Here's how the part is built. I have some questions about the finished solid (model axes, mm). A direction names the side the tool comes from. Round coordinates to 2 decimals unless told otherwise and drop trailing zeros. Write each loop counter-clockwise with the first axis right and the second up, starting at its lowest first coordinate (ties: lowest second). Pieces come first, ordered by that corner, then holes. Notation, with made-up numbers: M 56,47.25 L 106,47.25 A7 cw 106,59.25 Z; hole C 72,42.5 d10. An arc over 180 degrees is marked long. Use one line per item in the form item = value. Start each with the question number.
Q1. I need wall thicknesses on line 1 along X through (y, z) = (2.2, 14); line 2 along Z through (x, y) = (72, 2.25); line 3 along X through (y, z) = (2.85, 57). Which ranges of each line are inside material? Lowest first, please. Write a range as from..to.
Q2. I want a section at D-D on x = 72. List the corners of the cut face in (y, z) for me, and give its area (3 significant figures).
Q3. I want a section at C-C on z = 14. List the corners of the cut face in (x, y) for me, and give its area (3 significant figures).
Q4. We'd pull the mould along Z, two halves only. Please class faces 6 (the face through (41.243, 9.93, -20.533)), 7 (the face through (28.33, 2.535, 58.617)), 8 (the face through (63, 0, -44)): +Z half, -Z half, draft (parallel to the pull), parting line (faces both ways), or undercut.
Q5. For faces 1 (the face through (-43, 3, 40)), 2 (the face through (51, 10, -30)), 3 (the face through (-37, 3, 24.2)), 4 (the face through (-1, 0, -1)), 5 (the face through (-1, 5, -1)), which set-ups out of +Z, -Z, +X, -X, +Y, -Y let a thin tool reach every point of the face, with its end or its side?
Q6. I'm going to push flat-ended pins straight in: pin 1 Ø1.5 at (y, z) = (13, -40) entering from +X; pin 2 Ø8 at (y, z) = (7.5, 21.5) entering from +X; pin 3 Ø3 at (y, z) = (10.5, -28) entering from -X; pin 4 Ø8 at (x, z) = (-45, 11.5) entering from +Y. Where does each tip first touch, or does it pass through?
Q7. I want a section at A-A on y = 2.25. State how many separate pieces and enclosed holes the cut face has, and give its area (3 significant figures).
Q8. I want a section at B-B on x = -72. List the corners of the cut face in (y, z) for me, and give its area (4 significant figures).
```python
from build123d import *

# Parameters (mm, degrees)
SKETCH_2_W          = 150
SKETCH_2_H          = 120
EXTRUDE_1_DEPTH     = 5
SKETCH_3_R          = 1.65
SKETCH_3_R_2        = 1.75
CUT_EXTRUDE_1_DEPTH = 5
EXTRUDE_3_DEPTH     = 5
EXTRUDE_4_DEPTH     = 5
CUT_EXTRUDE_START   = -5
CUT_EXTRUDE_2_DEPTH = 5
CUT_EXTRUDE_4_DEPTH = 20
CUT_EXTRUDE_5_DEPTH = 10


with BuildPart() as part:
    # 草图2 → 凸台-拉伸1 (new body)
    with BuildSketch(Plane(origin=(0, 0, 0), x_dir=(1, 0, 0), z_dir=(0, 1, 0))):
        Rectangle(SKETCH_2_W, SKETCH_2_H)
    extrude(amount=EXTRUDE_1_DEPTH)

    # 草图3 → 切除-拉伸1 (cut)
    with BuildSketch(Plane(origin=(0, 5, 0), x_dir=(1, 0, 0), z_dir=(0, 1, 0))):
        with Locations(Location((-72, 57, 0), (0, 0, 270))):
            Circle(SKETCH_3_R)
        with Locations(Location((10, 57, 0), (0, 0, 270))):
            Circle(SKETCH_3_R)
        with Locations(Location((72, -57, 0), (0, 0, 270))):
            Circle(SKETCH_3_R_2)
        with Locations(Location((29, -57, 0), (0, 0, 270))):
            Circle(SKETCH_3_R_2)
        with Locations(Location((72, -14, 0), (0, 0, 270))):
            Circle(SKETCH_3_R_2)
        with Locations(Location((29, -14, 0), (0, 0, 270))):
            Circle(SKETCH_3_R_2)
        with BuildLine():
            Line((-43.138351407, -24.2), (-31.138351407, -24.2))
            ThreePointArc((-31.138351407, -24.2), (-29.338351407, -26), (-31.138351407, -27.8))
            Line((-31.138351407, -27.8), (-43.138351407, -27.8))
            ThreePointArc((-43.138351407, -27.8), (-44.938351407, -26), (-43.138351407, -24.2))
        make_face()
    extrude(amount=-CUT_EXTRUDE_1_DEPTH, mode=Mode.SUBTRACT)

    # 草图4 → 凸台-拉伸3 (add)
    with BuildSketch(Plane(origin=(0, 5, 0), x_dir=(1, 0, 0), z_dir=(0, 1, 0))):
        with BuildLine():
            Line((75, 24.250176471), (75, 60))
            Line((75, 60), (48.273565588, 60))
            ThreePointArc((48.273565588, 60), (59.086332475, 40.218381113), (75, 24.250176471))
        make_face()
        with BuildLine():
            Line((75, -6.509258806), (75, 0.045238901))
            ThreePointArc((75, 0.045238901), (44.912530325, 25.211568901), (26.791684351, 60))
            Line((26.791684351, 60), (20.764976647, 60))
            ThreePointArc((20.764976647, 60), (40.850679022, 21.0112766), (75, -6.509258806))
        make_face()
    extrude(amount=EXTRUDE_3_DEPTH)

    # 草图5 → 凸台-拉伸4 (add)
    with BuildSketch(Plane(origin=(0, 10, 0), x_dir=(1, 0, 0), z_dir=(0, 1, 0))):
        with BuildLine():
            Line((20.764976647, 60), (75, 60))
            Line((75, 60), (75, -6.509258806))
            ThreePointArc((75, -6.509258806), (40.850679022, 21.0112766), (20.764976647, 60))
        make_face()
    extrude(amount=EXTRUDE_4_DEPTH)

    # 草图6 → 切除-拉伸2 (cut)
    with BuildSketch(Plane(origin=(0, 5, 0), x_dir=(1, 0, 0), z_dir=(0, 1, 0)).offset(CUT_EXTRUDE_START)):
        with BuildLine():
            Line((48.273565588, 60), (26.791684351, 60))
            ThreePointArc((26.791684351, 60), (44.912530325, 25.211568901), (75, 0.045238901))
            Line((75, 0.045238901), (75, 24.250176471))
            ThreePointArc((75, 24.250176471), (59.086332475, 40.218381113), (48.273565588, 60))
        make_face()
    extrude(amount=CUT_EXTRUDE_2_DEPTH, mode=Mode.SUBTRACT)

    # 草图7 → 切除-拉伸4 (cut)
    with BuildSketch(Plane.XZ):
        with BuildLine():
            ThreePointArc((56.884646261, -60), (56.310021612, -61.397616975), (55.764937458, -62.807017544))
            Line((55.764937458, -62.807017544), (81.923412231, -71.445579772))
            Line((81.923412231, -71.445579772), (79.812030075, -30.641136223))
            ThreePointArc((79.812030075, -30.641136223), (77.363002414, -32.56982364), (75, -34.602996339))
            Line((75, -34.602996339), (75, -60))
            Line((75, -60), (56.884646261, -60))
        make_face()
        with BuildLine():
            ThreePointArc((75, -34.602996339), (64.546339392, -46.305761051), (56.884646261, -60))
            Line((56.884646261, -60), (75, -60))
            Line((75, -60), (75, -34.602996339))
        make_face()
    extrude(amount=-CUT_EXTRUDE_4_DEPTH, mode=Mode.SUBTRACT)

    # 草图8 → 切除-拉伸5 (cut)
    with BuildSketch(Plane(origin=(0, 5, 0), x_dir=(1, 0, 0), z_dir=(0, 1, 0))):
        with BuildLine():
            Line((-75, -40), (-10, -40))
            ThreePointArc((-10, -40), (10, -60), (-10, -80))
            Line((-10, -80), (-75, -80))
            ThreePointArc((-75, -80), (-95, -60), (-75, -40))
        make_face()
    extrude(amount=-CUT_EXTRUDE_5_DEPTH, mode=Mode.SUBTRACT)


solid = part.part
```
Reported:
q1.line_1 = -75..27.25, 30.75..70.25, 73.75..75
q1.line_2 = -37.46..-26.62, -1.75..12.25, 15.75..55.25, 58.75..60
q1.line_3 = 9.77..27.25, 30.75..70.25, 73.75..75
q2.outline = M 0,-37.46 L 15,-37.46 L 15,4.92 L 5,4.92 L 5,12.25 L 0,12.25 L 0,-1.75 L 10,-1.75 L 10,-26.62 L 0,-26.62 Z; M 0,15.75 L 5,15.75 L 5,55.25 L 0,55.25 Z; M 0,58.75 L 5,58.75 L 5,60 L 0,60 Z
q2.area = 627 mm^2
q3.outline = M -75,0 L 27.25,0 L 27.25,5 L -75,5 Z; M 30.75,0 L 70.25,0 L 70.25,5 L 30.75,5 Z; M 73.75,0 L 75,0 L 75,5 L 73.75,5 Z
q3.area = 715 mm^2
q4.face_6 = +Z half
q4.face_7 = undercut
q4.face_8 = draft
q5.face_1 = +Z, -X, +Y, -Y
q5.face_2 = -Y
q5.face_3 = +Y, -Y
q5.face_4 = +Z, -Z, +X, -X, -Y
q5.face_5 = +Z, -X, +Y
q6.pin_1 = 70.29
q6.pin_2 = 75
q6.pin_3 = 34.6
q6.pin_4 = 5
q7.separate_pieces = 2
q7.enclosed_holes = 7
q7.area = 14,700 mm^2
q8.outline = M 0,-60 L 5,-60 L 5,-58.65 L 0,-58.65 Z; M 0,-55.35 L 5,-55.35 L 5,40 L 0,40 Z
q8.area = 483.5 mm^2
